Could you check a few things on this model? Use its own coordinates, in mm. A direction names the side the tool comes from. Coordinates: 2 decimals unless noted, no trailing zeros. Write each loop counter-clockwise with the first axis right and the second up, starting at its lowest first coordinate (ties: lowest second). Pieces come first, ordered by that corner, then holes. Notation, with made-up numbers: (-20.75, 57) - (23.25, 57) arc R14 cw to (23.25, 79) - close; hole circle Ø10 at (74, 27). An arc over 180 degrees is marked (long way). Write item = value, one per line. Start each with the question number.
```python
from build123d import *

# Parameters (mm, degrees)
F0_R     = 31.1
F1_DEPTH = 3
F2_SIZE  = 2
F3_R     = 26
F4_DEPTH = 16
F5_R     = 2
F6_W     = 1
F6_H     = 8
F7_DEPTH = 13


with BuildPart() as f1:
    # F0 (on Top) → F1 (new body)
    with BuildSketch(Plane.XY):
        Circle(F0_R)
    extrude(amount=F1_DEPTH)

    # F2
    f2_edges = [f1.edges().sort_by_distance(p)[0] for p in [
        (-31.1, 0, 3),
    ]]
    chamfer(f2_edges, length=F2_SIZE)

    # F3 (on face) → F4 (join)
    with BuildSketch(Plane(origin=(0, 0, 0), x_dir=(1, 0, 0), z_dir=(0, 0, -1))):
        Circle(F3_R)
    extrude(amount=F4_DEPTH)

    # F5
    f5_edges = [f1.edges().sort_by_distance(p)[0] for p in [
        (-26, 0, -16),
    ]]
    fillet(f5_edges, radius=F5_R)

    # F6 (on face) → F7 (join)
    with BuildSketch(Plane(origin=(0, 0, -16), x_dir=(1, 0, 0), z_dir=(0, 0, -1))):
        with Locations((-20.5, 0)):
            Rectangle(F6_W, F6_H)
        with Locations((20.5, 0)):
            Rectangle(F6_W, F6_H)
    extrude(amount=F7_DEPTH)

    # F9 (on Front) → F10 (revolve)
    with BuildSketch(Plane.XZ):
        with BuildLine():
            Line((-23.5, 3), (0, 3))
            Line((0, 3), (0, 14))
            add(Edge.make_bspline(
                [(-23.5, 3), (-23.5445970751, 5.3470100891), (-23.3472398778, 11.6386271394), (-3.4499369243, 14.3252252988), (-0.5936216616, 14), (0, 14)],
                knots=[0, 0, 0, 0, 0.3018049736, 0.7936654017, 1, 1, 1, 1], degree=3))
        make_face()
    revolve(axis=Axis((0, 0, 8.5), (0, 0, 1)))


solid = f1.part
```
1) If I drill on probe 1 along X at (y, z) = (0.5, -5.5); probe 2 along Z at (x, y) = (18.5, 15); probe 3 along X at (y, z) = (13.5, -14.5), over which ranges is the centre line in solid material (lowest first)? Write a range as [from, to].
2) Thinking about a two-plate mould opening in X: for faces 1 (the cylindrical face through (-6.74, -30.36, 0.49)), 2 (the flat face through (-7.1, -25.2, 0)), 3 (the flat face through (20, 0, -22)), 4 (the flat face through (-20, 0, -22)), which applies, +X half, -X half, draft (parallel to the pull), parting line (faces both ways), or undercut?
3) For P1, Ø0.5, axis at x = -20.5, z = -20, coming from the -Y side; P2, Ø10, axis at x = 2.5, z = -12, coming from the +Y side; P3, Ø1.5, axis at x = 11, z = -14, coming from the +Y side, each with a flat end and sliding along its axis, tell me the tip position at first contact or that it passes through.
4) Which directions (+Z, -Z, +X, -X, +Y, -Y) give clear straight access to the entire face, cutting with the end or side of a thin tool? Please do faces 5 (the flat face through (21, 0, -22)), 6 (the cylindrical face through (-20.633, 15.821, -6.902)), 7 (the flat face through (-21, 0, -22)).
5) Suppose I cut it at A-A on z = -10. Please give me the cut outline in (x, y), plus the area to 3 significant figures.
Reply:
q1.probe_1 = [-26, 26]
q1.probe_2 = [-16, 3]
q1.probe_3 = [-22.15, 22.15]
q2.face_1 = parting line
q2.face_2 = draft
q2.face_3 = undercut
q2.face_4 = undercut
q3.P1 = -4
q3.P2 = 26
q3.P3 = 23.89
q4.face_5 = -Z, +X, +Y, -Y
q4.face_6 = -Z
q4.face_7 = -Z, -X, +Y, -Y
q5.outline = circle Ø52 at (0, 0)
q5.area = 2,120 mm^2
